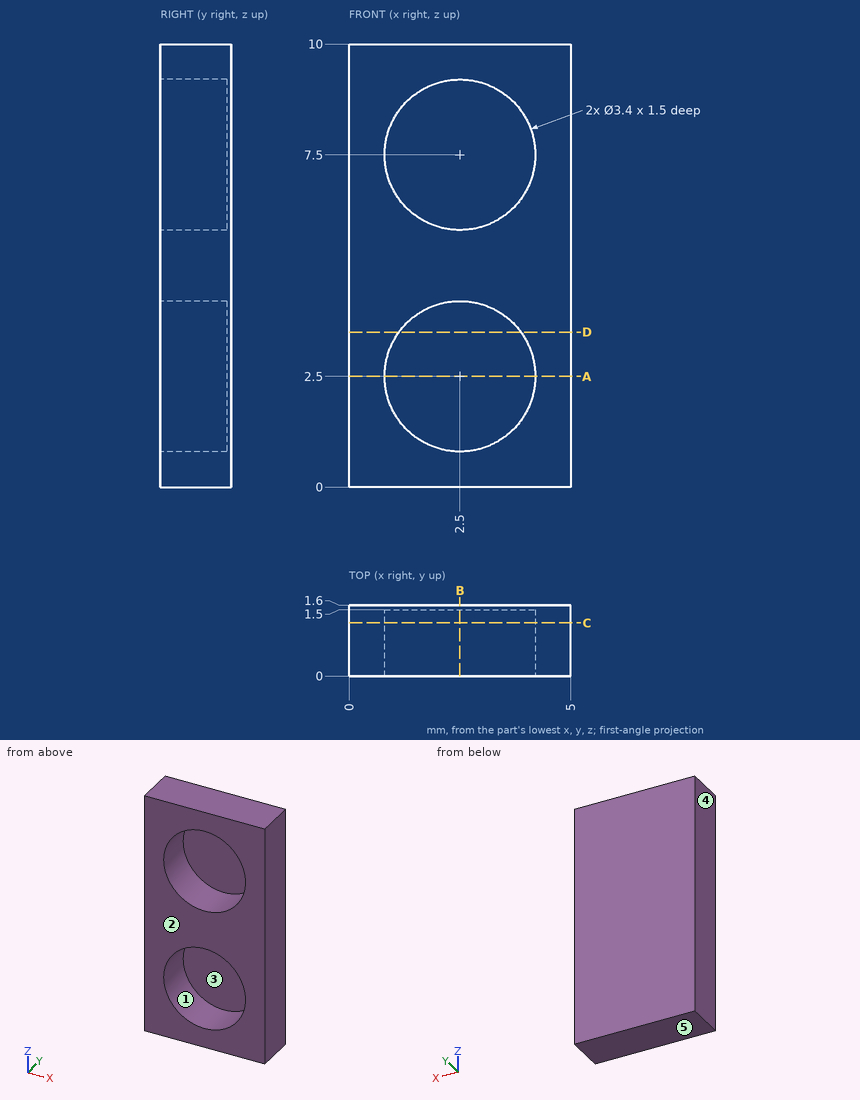
Drawing for the job (mm, zero at the part's lowest x, y, z). A direction names the side the tool comes from. Round coordinates to 2 decimals unless told otherwise and drop trailing zeros. Write each loop counter-clockwise with the first axis right and the second up, starting at its lowest first coordinate (ties: lowest second). Pieces come first, ordered by that corner, then holes. Notation, with made-up numbers: M -18,81.25 L -14,81.25 A12 ccw -14,100.25 Z; hole C 89.5,-34.5 d1. An arc over 180 degrees is marked long. Answer in a Markdown table with one row per item.
1. Saw through at B-B (x = 2.5). List the corners of the cut face in (y, z), and give its area (3 significant figures).
Geometry check:
| item | result |
|---|---|
| outline | M 0,0 L 1.6,0 L 1.6,10 L 0,10 L 0,9.2 L 1.5,9.2 L 1.5,5.8 L 0,5.8 L 0,4.2 L 1.5,4.2 L 1.5,0.8 L 0,0.8 Z |
| area | 5.80 mm2 |
2. Mould opens along Z. For the marked faces 3, 4 and 5 say: +Z half, -Z half, draft (parallel to the pull), parting line (faces both ways), or undercut.
Geometry check:
| item | result |
|---|---|
| face 3 | undercut |
| face 4 | draft |
| face 5 | -Z half |
3. Flat gauge pin, fed straight in: P1, Ø2, axis at x = 2.5, z = 2.5, coming from the -Y side. Where does the tip first touch, or does it go through?
Geometry check:
| item | result |
|---|---|
| P1 | y = 1.5 |
4. Which spindle directions (+Z, -Z, +X, -X, +Y, -Y) get a long thin tool onto all of the face, cutting with end or side? Do the marked faces 1 and 2. Say none if no direction does.
Geometry check:
| item | result |
|---|---|
| face 1 | -Y |
| face 2 | +Z, -Z, +X, -X, -Y |
5. Saw through at A-A (z = 2.5). List the corners of the cut face in (x, y).
Geometry check:
| item | result |
|---|---|
| outline | M 0,0 L 0.8,0 L 0.8,1.5 L 4.2,1.5 L 4.2,0 L 5,0 L 5,1.6 L 0,1.6 Z |
6. Saw through at C-C (y = 1.2). List the corners of the cut face in (x, z), and give its area (3 significant figures).
Geometry check:
| item | result |
|---|---|
| outline | M 0,0 L 5,0 L 5,10 L 0,10 Z; hole C 2.5,2.5 d3.4; hole C 2.5,7.5 d3.4 |
| area | 31.8 mm2 |
7. Saw through at D-D (z = 3.5). List the corners of the cut face in (x, y).
Geometry check:
| item | result |
|---|---|
| outline | M 0,0 L 1.13,0 L 1.13,1.5 L 3.87,1.5 L 3.87,0 L 5,0 L 5,1.6 L 0,1.6 Z |
8. Probe L1, parallel to Z at x = 2.6, y = 0.9; L2, parallel to Z at x = 2.05, y = 0.2; L3, parallel to X at y = 0.8, z = 7.75. List the from-to ranges inside material, lowest first. Write a range as [from, to].
Geometry check:
| item | result |
|---|---|
| L1 | [0, 0.8], [4.2, 5.8], [9.2, 10] |
| L2 | [0, 0.86], [4.14, 5.86], [9.14, 10] |
| L3 | [0, 0.82], [4.18, 5] |
